Verification items for the finished model (mm, model axes). Face numbers are marked on the shaded views. Give positions to 0.01 mm unless a question says otherwise; leave off trailing zeros. Loops run counter-clockwise (first coordinate to the right, second up) from the corner with the lowest first, then second, coordinate; pieces in that order, holes last. Notation, with made-up numbers: (-17, 51) - (36, 51) arc R12 cw to (36, 64) - close; hole circle Ø9 at (19, 30). An arc over 180 degrees is marked (long way). Answer in a Markdown table with one row per item.
```python
from build123d import *

# Parameters (mm, degrees)
SKETCH1_R           = 4.5
SKETCH1_R_2         = 2.5
BOSS_EXTRUDE1_DEPTH = 22.5
CHAMFER1_SIZE       = 0.5


with BuildPart() as part:
    # Sketch1 → Boss-Extrude1 (new, symmetric)
    with BuildSketch(Plane.XY):
        with Locations(Location((0, 0, 0), (0, 0, 180))):
            Circle(SKETCH1_R)
        with Locations(Location((0, 0, 0), (0, 0, 180))):
            Circle(SKETCH1_R_2, mode=Mode.SUBTRACT)
    extrude(amount=BOSS_EXTRUDE1_DEPTH, both=True)

    # Chamfer1
    chamfer1_edges = [part.edges().sort_by_distance(p)[0] for p in [
        (4.5, 0, -22.5),
        (4.5, 0, 22.5),
        (2.5, 0, -22.5),
        (2.5, 0, 22.5),
    ]]
    chamfer(chamfer1_edges, length=CHAMFER1_SIZE)


solid = part.part
```
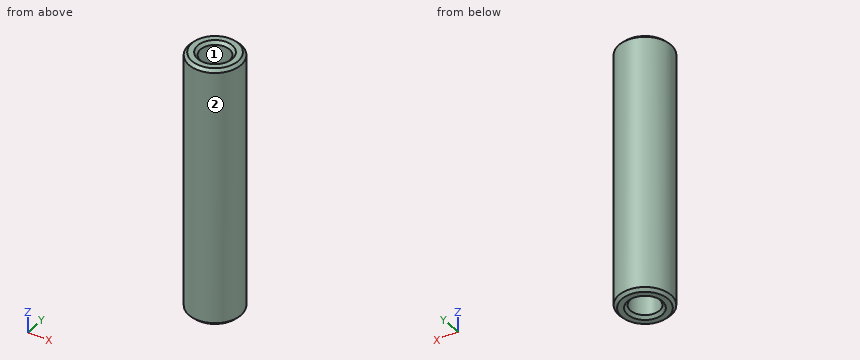
Q1. Sectioned sample at A-A (y = 0). Record the cut outline in (x, z), and give its area (3 significant figures).
Completed:
| item | result |
|---|---|
| outline | (-4.5, -22) - (-4, -22.5) - (-3, -22.5) - (-2.5, -22) - (-2.5, 22) - (-3, 22.5) - (-4, 22.5) - (-4.5, 22) - close; (2.5, -22) - (3, -22.5) - (4, -22.5) - (4.5, -22) - (4.5, 22) - (4, 22.5) - (3, 22.5) - (2.5, 22) - close |
| area | 179 mm^2 |
Q2. Go/stop test with flat-tipped pins: P1, Ø2, axis at x = -2, z = -7.5, coming from the -Y side; P2, Ø5, axis at x = -3, y = 3, coming from the +Z side; P3, Ø3, axis at y = 3, z = 11, coming from the +X side. Record where each tip stops, or that it passes through.
Completed:
| item | result |
|---|---|
| P1 | y = -4.39 |
| P2 | z = 22.5 |
| P3 | x = 4.24 |
Q3. Draft check along X on the marked faces 1 and 2. Enter one of: +X half, -X half, draft (parallel to the pull), parting line (faces both ways), or undercut.
Completed:
| item | result |
|---|---|
| face 1 | undercut |
| face 2 | parting line |
Q4. Thickness scan on line 1 (Y direction, x = 0, z = 9); line 2 (X direction, y = -0.25, z = -9); line 3 (X direction, y = -2.25, z = 4). Record the ranges inside material, lowest first.
Completed:
| item | result |
|---|---|
| line 1 | -4.5 to -2.5, 2.5 to 4.5 |
| line 2 | -4.49 to -2.49, 2.49 to 4.49 |
| line 3 | -3.9 to -1.09, 1.09 to 3.9 |
Q5. Sectioned sample at C-C (z = 5). Record the cut outline in (x, y).
Completed:
| item | result |
|---|---|
| outline | circle Ø9 at (0, 0); hole circle Ø5 at (0, 0) |
